```python
from build123d import *

# Parameters (mm, degrees)
F0_W        = 264.5
F0_H        = 7.2
F0_R        = 1
F0_R_2      = 2.75
F1_DEPTH    = 3
F2_T1_DEPTH = 269.6433659759


# Not quite as in the source:
# - a fillet or chamfer that OpenCascade refuses, or shapes differently, is made with other operations: its cross-section is extruded or revolved along the edge and cut away or added


with BuildPart() as f1:
    # F0 (on Front) → F1 (new body)
    with BuildSketch(Plane.XZ):
        Rectangle(F0_W, F0_H)
        with Locations((-113.25, -2.1)):
            Circle(F0_R, mode=Mode.SUBTRACT)
        with Locations((-109.5, 0)):
            Circle(F0_R_2, mode=Mode.SUBTRACT)
        with Locations((-84.5, 0)):
            Circle(F0_R_2, mode=Mode.SUBTRACT)
        with Locations((-59.5, 0)):
            Circle(F0_R_2, mode=Mode.SUBTRACT)
        with Locations((-34.5, 0)):
            Circle(F0_R_2, mode=Mode.SUBTRACT)
        with Locations((-9.5, 0)):
            Circle(F0_R_2, mode=Mode.SUBTRACT)
        with Locations((-113.25, 2.1)):
            Circle(F0_R, mode=Mode.SUBTRACT)
        with Locations((15.5, 0)):
            Circle(F0_R_2, mode=Mode.SUBTRACT)
        with Locations((40.5, 0)):
            Circle(F0_R_2, mode=Mode.SUBTRACT)
        with Locations((65.5, 0)):
            Circle(F0_R_2, mode=Mode.SUBTRACT)
        with Locations((90.5, 0)):
            Circle(F0_R_2, mode=Mode.SUBTRACT)
        with Locations((115.5, 0)):
            Circle(F0_R_2, mode=Mode.SUBTRACT)
    extrude(amount=F1_DEPTH)

    # F2: chamfer of 1 on 4 edges, made by hand

    # F2_s2 → F2_t1 (cut)
    with BuildSketch(Plane.YZ.offset(-134.821682988)):
        Polygon((-2, -3.6), (-3, -2.6), (-3, -3.6), align=None)
        Polygon((-1, -3.6), (0, -2.6), (0, -3.6), align=None)
        Polygon((-1, 3.6), (0, 2.6), (0, 3.6), align=None)
        Polygon((-2, 3.6), (-3, 2.6), (-3, 3.6), align=None)
    extrude(amount=F2_T1_DEPTH, mode=Mode.SUBTRACT)


solid = f1.part
```
Source: CAD feature listing. Evaluate the final solid. Frame: model axes, mm. Round coordinates to 2 decimals unless told otherwise and drop trailing zeros. Loops run counter-clockwise (first coordinate to the right, second up) from the corner with the lowest first, then second, coordinate; pieces in that order, holes last.
1. Mould query, pull axis Z, two halves, no side actions, for faces 1 (the cylindrical face through (-6.96, -1.48, -1.05)), 2 (the flat face through (-121, -3, 0)). Classes: released by +Z, released by -Z, zero draft, split by the parting line, or undercut.
2. Section query A-A on x = 73. Output: boundary loops of the cut face in (y, z).
3. Ray query, L1, parallel to Z at x = 15.5, y = -1.4; L2, parallel to Z at x = -5, y = -2.5; L3, parallel to X at y = -1.15, z = 3. Return the intervals inside material, ascending.
Answers below:
1. face 1: undercut
1. face 2: zero draft
2. outline: (-3, -2.6) - (-2, -3.6) - (-1, -3.6) - (0, -2.6) - (0, 2.6) - (-1, 3.6) - (-2, 3.6) - (-3, 2.6) - close
3. L1: z = -3.6 to -2.75, 2.75 to 3.6
3. L2: z = -3.1 to 3.1
3. L3: x = -132.25 to -113.69, -112.81 to 132.25
